```python
from build123d import *

# Parameters (mm, degrees)
SKETCH1_W           = 38.1
SKETCH1_H           = 20.32
BOSS_EXTRUDE1_DEPTH = 0.7874
SKETCH3_R           = 1.65
CUT_EXTRUDE2_DEPTH  = 10
SKETCH4_R           = 6
BOSS_EXTRUDE2_DEPTH = 8
FILLET1_R           = 1
SKETCH5_R           = 1.2
CUT_EXTRUDE3_DEPTH  = 2
SKETCH6_W           = 11
SKETCH6_H           = 14
BOSS_EXTRUDE3_DEPTH = 12
CUT_EXTRUDE4_DEPTH  = 12
SKETCH8_R           = 1
CUT_EXTRUDE5_DEPTH  = 1
SKETCH9_W           = 4.608332255
SKETCH9_H           = 6.248586108
SKETCH9_W_2         = 4.008332255
SKETCH9_H_2         = 5.648586108
BOSS_EXTRUDE4_DEPTH = 8


with BuildPart() as part:
    # Sketch1 → Boss-Extrude1 (new body)
    with BuildSketch(Plane(origin=(0, 0, 0), x_dir=(1, 0, 0), z_dir=(0, 1, 0))):
        Rectangle(SKETCH1_W, SKETCH1_H)
    extrude(amount=BOSS_EXTRUDE1_DEPTH)

    # Sketch3 → Cut-Extrude2 (cut)
    with BuildSketch(Plane.XZ):
        with Locations(Location((-15.7, 7, 0), (0, 0, 270))):
            Circle(SKETCH3_R)
        with Locations(Location((15.7, 7, 0), (0, 0, 270))):
            Circle(SKETCH3_R)
        with Locations(Location((15.7, -7, 0), (0, 0, 270))):
            Circle(SKETCH3_R)
        with Locations(Location((-15.7, -7, 0), (0, 0, 270))):
            Circle(SKETCH3_R)
    extrude(amount=-CUT_EXTRUDE2_DEPTH, mode=Mode.SUBTRACT)

    # Sketch4 → Boss-Extrude2 (add)
    with BuildSketch(Plane(origin=(0, 0.7874, 0), x_dir=(1, 0, 0), z_dir=(0, 1, 0))):
        with Locations(Location((-10, 0, 0), (0, 0, 270))):
            Circle(SKETCH4_R)
    extrude(amount=BOSS_EXTRUDE2_DEPTH)

    # Fillet1
    fillet1_edges = [part.edges().sort_by_distance(p)[0] for p in [
        (-10, 8.7874, -6),
    ]]
    fillet(fillet1_edges, radius=FILLET1_R)

    # Sketch5 → Cut-Extrude3 (cut)
    with BuildSketch(Plane(origin=(0, 8.7874, 0), x_dir=(1, 0, 0), z_dir=(0, 1, 0))):
        with Locations(Location((-10, 0, 0), (0, 0, 270))):
            Circle(SKETCH5_R)
    extrude(amount=-CUT_EXTRUDE3_DEPTH, mode=Mode.SUBTRACT)

    # Sketch6 → Boss-Extrude3 (add)
    with BuildSketch(Plane(origin=(0, 0.7874, 0), x_dir=(1, 0, 0), z_dir=(0, 1, 0))):
        with Locations((6.7, 0.5)):
            Rectangle(SKETCH6_W, SKETCH6_H)
    extrude(amount=BOSS_EXTRUDE3_DEPTH)

    # Sketch7 → Cut-Extrude4 (cut)
    with BuildSketch(Plane(origin=(12.2, 0, 0), x_dir=(0, 0, -1), z_dir=(1, 0, 0))):
        Polygon((-6, 7.7874), (-4.984156555, 12.7874), (-6.5, 12.7874), (-6.5, 7.7874), align=None)
        Polygon((-1.984156555, 12.7874), (-0.96831311, 7.7874), (1.96831311, 7.7874), (2.984156555, 12.7874), align=None)
        Polygon((5.984156555, 12.7874), (7, 7.7874), (7.5, 7.7874), (7.5, 12.7874), align=None)
    extrude(amount=-CUT_EXTRUDE4_DEPTH, mode=Mode.SUBTRACT)

    # Sketch8 → Cut-Extrude5 (cut)
    with BuildSketch(Plane(origin=(0, 12.7874, 0), x_dir=(1, 0, 0), z_dir=(0, 1, 0))):
        with Locations(Location((10.75, -3.484156555, 0), (0, 0, 270))):
            Circle(SKETCH8_R)
        with Locations(Location((8.05, -3.484156555, 0), (0, 0, 270))):
            Circle(SKETCH8_R)
        with Locations(Location((5.35, -3.484156555, 0), (0, 0, 270))):
            Circle(SKETCH8_R)
        with Locations(Location((2.65, -3.484156555, 0), (0, 0, 270))):
            Circle(SKETCH8_R)
        with Locations(Location((10.75, 4.484156555, 0), (0, 0, 270))):
            Circle(SKETCH8_R)
        with Locations(Location((8.05, 4.484156555, 0), (0, 0, 270))):
            Circle(SKETCH8_R)
        with Locations(Location((5.35, 4.484156555, 0), (0, 0, 270))):
            Circle(SKETCH8_R)
        with Locations(Location((2.65, 4.484156555, 0), (0, 0, 270))):
            Circle(SKETCH8_R)
    extrude(amount=-CUT_EXTRUDE5_DEPTH, mode=Mode.SUBTRACT)

    # Sketch9 → Boss-Extrude4 (add)
    with BuildSketch(Plane(origin=(0, 0.7874, 0), x_dir=(1, 0, 0), z_dir=(0, 1, 0))):
        with Locations((16.246323881, 0.234321979)):
            Rectangle(SKETCH9_W, SKETCH9_H)
        with Locations((16.246323881, 0.234321979)):
            Rectangle(SKETCH9_W_2, SKETCH9_H_2, mode=Mode.SUBTRACT)
    extrude(amount=BOSS_EXTRUDE4_DEPTH)


solid = part.part
```
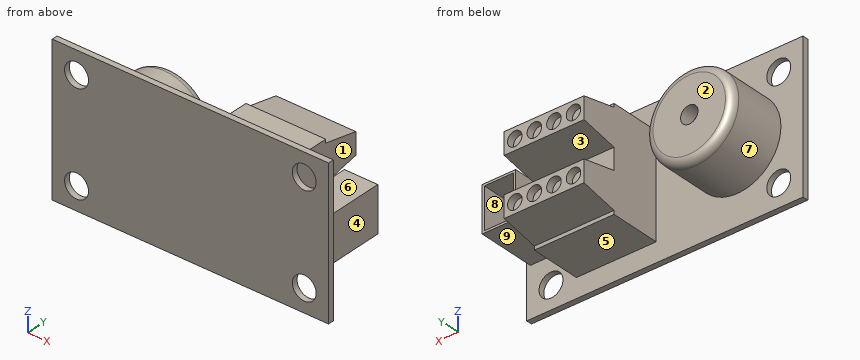
Design review of the part built by this model. Coordinates are the model's own, in mm. Face numbers are marked on the shaded views. A direction names the side the tool comes from. Give positions to 0.01 mm unless a question says otherwise; leave off trailing zeros. Loops run counter-clockwise (first coordinate to the right, second up) from the corner with the lowest first, then second, coordinate; pieces in that order, holes last. Notation, with made-up numbers: (-34, 61.25) -> (8, 61.25) arc R19 cw to (8, 87.25) -> close; hole circle Ø6 at (-2.5, 39). An arc over 180 degrees is marked (long way). One line per item, written item: value.
Q1. Draft analysis for pull direction Z (two halves, no side actions). For the marked faces 6, 7, 8 and 9, state which applies: pulls with the +Z half, pulls with the -Z half, needs draft (parallel to the pull), parting line crosses it, or undercut.
Numbers:
face 6: pulls with the +Z half
face 7: parting line crosses it
face 8: undercut
face 9: pulls with the -Z half
Q2. We need section A-A on z = 7. Give the boundary of the cut face in (x, y), and give its area (3 significant figures).
Numbers:
outline: (-19.05, 0) -> (-17.35, 0) -> (-17.35, 0.79) -> (-19.05, 0.79) -> close; (-14.05, 0) -> (14.05, 0) -> (14.05, 0.79) -> (-14.05, 0.79) -> close; (17.35, 0) -> (19.05, 0) -> (19.05, 0.79) -> (17.35, 0.79) -> close
area: 24.8 mm^2
Q3. For L1, parallel to X at y = 0.65, z = -7; L2, parallel to X at y = 8.3, z = 0; L3, parallel to X at y = 8.25, z = -6, list the stretches that pass through material, from the lowest coordinate up.
Numbers:
L1: x = -19.05 to -17.35, -14.05 to 14.05, 17.35 to 19.05
L2: x = -15.86 to -11.2, -8.8 to -4.14, 13.94 to 14.24, 18.25 to 18.55
L3: x = 1.2 to 12.2
Q4. We need section B-B on y = 12.25. Give the number of separate pieces and of enclosed holes in the cut face, and give its area (3 significant figures).
Numbers:
separate pieces: 2
enclosed holes: 8
area: 45.7 mm^2
Q5. Machinability: for the marked faces 1, 2, 3, 4 and 5, which of the approach directions +Z, -Z, +X, -X, +Y, -Y give a long, thin tool a straight path to every point of the face, cutting with its end or side? Answer none if there is none.
Numbers:
face 1: +Z, -Z, +Y
face 2: +Z, -Z, -X, +Y
face 3: +Y
face 4: +Z, -Z, +X, +Y
face 5: -Z, +X, -X, +Y
Q6. For pin 1 Ø0.6 at (x, z) = (11, 4) entering from +Y; pin 2 Ø4.5 at (x, z) = (15.7, -7) entering from -Y; pin 3 Ø3.5 at (x, y) = (8, 4) entering from +Z; pin 4 Ø5 at (y, z) = (5.5, 7) entering from -X, all flat-tipped, find the tip position at first contact; note any pin that passes through.
Numbers:
pin 1: stops at y = 11.79
pin 2: stops at y = 0
pin 3: stops at z = 6.5
pin 4: stops at x = -13.97
Q7. We need section D-D on z = 0. Give the boundary of the cut face in (x, y), and give its area (3 significant figures).
Numbers:
outline: (-19.05, 0) -> (19.05, 0) -> (19.05, 0.79) -> (18.55, 0.79) -> (18.55, 8.79) -> (18.25, 8.79) -> (18.25, 0.79) -> (14.24, 0.79) -> (14.24, 8.79) -> (13.94, 8.79) -> (13.94, 0.79) -> (12.2, 0.79) -> (12.2, 7.79) -> (1.2, 7.79) -> (1.2, 0.79) -> (-4, 0.79) -> (-4, 7.79) arc R1 ccw to (-5, 8.79) -> (-8.8, 8.79) -> (-8.8, 6.79) -> (-11.2, 6.79) -> (-11.2, 8.79) -> (-15, 8.79) arc R1 ccw to (-16, 7.79) -> (-16, 0.79) -> (-19.05, 0.79) -> close
area: 203 mm^2
Q8. We need section C-C on x = 16.5. Give the boundary of the cut face in (y, z), and give its area (3 significant figures).
Numbers:
outline: (0, -10.16) -> (0.79, -10.16) -> (0.79, -8.44) -> (0, -8.44) -> close; (0, -5.56) -> (0.79, -5.56) -> (0.79, -3.36) -> (8.79, -3.36) -> (8.79, -3.06) -> (0.79, -3.06) -> (0.79, 2.59) -> (8.79, 2.59) -> (8.79, 2.89) -> (0.79, 2.89) -> (0.79, 5.56) -> (0, 5.56) -> close; (0, 8.44) -> (0.79, 8.44) -> (0.79, 10.16) -> (0, 10.16) -> close
area: 16.3 mm^2
